CAD build for the part. Positions are in the model's coordinates, mm. Coordinates: 2 decimals unless noted, no trailing zeros. Order: outer loops, then holes, each group sorted by start corner. A loop starts at its lowest first (then second) coordinate and runs counter-clockwise, first axis right, second up. Notation, with made-up numbers: (57, -14.5) - (113, -14.5) arc R19 ccw to (113, 3.5) - close; hole circle Ø2 at (12.5, 63.5). An arc over 180 degrees is marked (long way). Use one line per item in the form item = value.
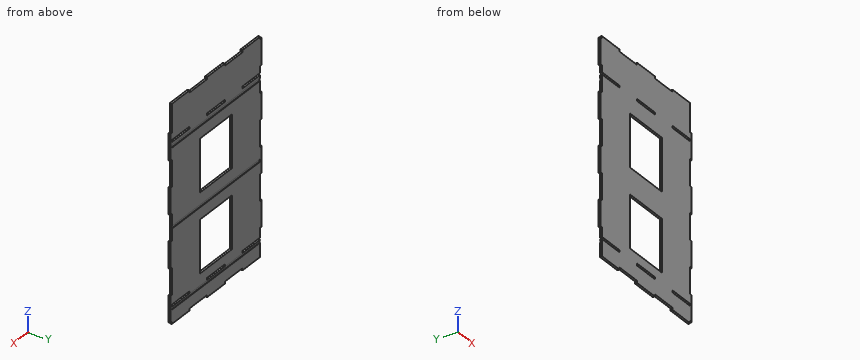
Autodesk Inventor part; units mm, degrees
ref_plane "YZ Plane" through (0, 0, 0) normal (1, 0, 0) x (0, 1, 0)
ref_plane "XZ Plane" through (0, 0, 0) normal (0, 1, 0) x (-1, 0, 0)
ref_plane "XY Plane" through (0, 0, 0) normal (0, 0, 1) x (1, 0, 0)
sketch "Sketch1" plane through (0, 0, 0) normal (0, 1, 0) x (-1, 0, 0)
  line L0 (-125, 200) -> (125, 200) construction
  line L1 (125, 200) -> (125, -200) construction
  line L2 (125, -200) -> (-125, -200) construction
  line L3 (-125, -200) -> (-125, 200) construction
  line L4 (-125, 200) -> (125, -200) construction
  line L5 (125, 200) -> (-125, -200) construction
  line L6 (125, 200) -> (75, 200) construction
  line L7 (75, 200) -> (75, 204)
  line L8 (75, 204) -> (125, 204)
  line L9 (125, 204) -> (125, 200)
  line L10 (125, 200) -> (129, 200)
  line L11 (129, 200) -> (129, 150)
  line L12 (129, 150) -> (125, 150)
  line L13 (125, 150) -> (125, 200) construction
  line L14 (-125, 200) -> (-129, 200) construction
  line L15 (-129, 200) -> (-129, 150) construction
  line L16 (-129, 150) -> (-125, 150)
  line L17 (-125, 150) -> (-125, 200)
  line L18 (125, -200) -> (75, -200) construction
  line L19 (75, -200) -> (75, -204)
  line L20 (75, -204) -> (125, -204)
  line L21 (125, -204) -> (125, -200)
  line L22 (125, 100) -> (125, 150)
  line L23 (125, 150) -> (129, 150)
  line L24 (129, 100) -> (125, 100)
  line L25 (129, 150) -> (129, 100) construction
  line L26 (-125, 100) -> (-125, 150) construction
  line L27 (-125, 150) -> (-129, 150)
  line L28 (-129, 150) -> (-129, 100)
  line L29 (-129, 100) -> (-125, 100)
  line L30 (125, 50) -> (125, 100) construction
  line L31 (125, 100) -> (129, 100)
  line L32 (129, 50) -> (125, 50)
  line L33 (129, 100) -> (129, 50)
  line L34 (-125, 50) -> (-125, 100)
  line L35 (-125, 100) -> (-129, 100)
  line L36 (-129, 100) -> (-129, 50) construction
  line L37 (-129, 50) -> (-125, 50)
  line L38 (125, 0) -> (125, 50)
  line L39 (125, 50) -> (129, 50)
  line L40 (129, 0) -> (125, 0)
  line L41 (129, 50) -> (129, 0) construction
  line L42 (-125, 0) -> (-125, 50) construction
  line L43 (-125, 50) -> (-129, 50)
  line L44 (-129, 50) -> (-129, 0)
  line L45 (-129, 0) -> (-125, 0)
  line L46 (125, -50) -> (125, 0) construction
  line L47 (125, 0) -> (129, 0)
  line L48 (129, -50) -> (125, -50)
  line L49 (129, 0) -> (129, -50)
  line L50 (-125, -50) -> (-125, 0)
  line L51 (-125, 0) -> (-129, 0)
  line L52 (-129, 0) -> (-129, -50) construction
  line L53 (-129, -50) -> (-125, -50)
  line L54 (125, -100) -> (125, -50)
  line L55 (125, -50) -> (129, -50)
  line L56 (129, -100) -> (125, -100)
  line L57 (129, -50) -> (129, -100) construction
  line L58 (-125, -100) -> (-125, -50) construction
  line L59 (-125, -50) -> (-129, -50)
  line L60 (-129, -50) -> (-129, -100)
  line L61 (-129, -100) -> (-125, -100)
  line L62 (125, -150) -> (125, -100) construction
  line L63 (125, -100) -> (129, -100)
  line L64 (129, -150) -> (125, -150)
  line L65 (129, -100) -> (129, -150)
  line L66 (-125, -150) -> (-125, -100)
  line L67 (-125, -100) -> (-129, -100)
  line L68 (-129, -100) -> (-129, -150) construction
  line L69 (-129, -150) -> (-125, -150)
  line L70 (125, -200) -> (125, -150)
  line L71 (125, -150) -> (129, -150)
  line L72 (129, -200) -> (125, -200) construction
  line L73 (129, -150) -> (129, -200) construction
  line L74 (-125, -200) -> (-125, -150) construction
  line L75 (-125, -150) -> (-129, -150)
  line L76 (-129, -150) -> (-129, -200)
  line L77 (-129, -200) -> (-125, -200)
  line L78 (75, 204) -> (75, 200)
  line L79 (25, 200) -> (25, 204)
  line L80 (25, 204) -> (75, 204) construction
  line L81 (75, 200) -> (25, 200)
  line L82 (75, -200) -> (25, -200)
  line L83 (25, -200) -> (25, -204)
  line L84 (25, -204) -> (75, -204) construction
  line L85 (75, -204) -> (75, -200)
  line L86 (25, 204) -> (25, 200)
  line L87 (-25, 200) -> (-25, 204)
  line L88 (-25, 204) -> (25, 204)
  line L89 (25, 200) -> (-25, 200) construction
  line L90 (25, -200) -> (-25, -200) construction
  line L91 (-25, -200) -> (-25, -204)
  line L92 (-25, -204) -> (25, -204)
  line L93 (25, -204) -> (25, -200)
  line L94 (-25, 204) -> (-25, 200)
  line L95 (-75, 200) -> (-75, 204)
  line L96 (-75, 204) -> (-25, 204) construction
  line L97 (-25, 200) -> (-75, 200)
  line L98 (-25, -200) -> (-75, -200)
  line L99 (-75, -200) -> (-75, -204)
  line L100 (-75, -204) -> (-25, -204) construction
  line L101 (-25, -204) -> (-25, -200)
  line L102 (-75, 204) -> (-75, 200)
  line L103 (-125, 200) -> (-125, 204)
  line L104 (-125, 204) -> (-75, 204)
  line L105 (-75, 200) -> (-125, 200) construction
  line L106 (-75, -200) -> (-125, -200) construction
  line L107 (-125, -200) -> (-125, -204)
  line L108 (-125, -204) -> (-75, -204)
  line L109 (-75, -204) -> (-75, -200)
  point P0 (0, 0)
  dimension "d0" = 250
  dimension "d1" = 400
  dimension "d2" = 50
  dimension "d3" = 4
  dimension "d4" = 4
  dimension "d5" = 50
  dimension "d6" = 4
  dimension "d7" = 50
  dimension "d8" = 50
  dimension "d9" = 4
  dimension "d12" = 50
  dimension "d19" = 50
extrude "Extrusion1" add sketch "Sketch1" along normal blind 4
sketch "Sketch2" plane through (0, 4, 0) normal (0, 1, 0) x (1, 0, 0)
  line L0 (-125, 100) -> (-125, 50)
  line L1 (129, 100) -> (125, 100)
  line L2 (-125, 100) -> (125, 100) construction
  line L3 (125, -100) -> (125, -50)
  line L4 (125, -50) -> (-125, -50) construction
  line L5 (-45, 150) -> (45, 150)
  line L6 (45, 150) -> (45, 50)
  line L7 (45, 50) -> (-45, 50)
  line L8 (-45, 50) -> (-45, 150)
  line L9 (-45, 150) -> (45, 50) construction
  line L10 (45, 150) -> (-45, 50) construction
  line L11 (45, -100) -> (-45, -100)
  line L12 (-45, -100) -> (-45, 0)
  line L13 (-45, 0) -> (45, 0)
  line L14 (45, 0) -> (45, -100)
  line L15 (45, -100) -> (-45, 0) construction
  line L16 (-45, -100) -> (45, 0) construction
  point P0 (0, 0)
  point P1 (0, 100)
  point P2 (0, -50)
  point P3 (0, -50)
  dimension "d26" = 90
  dimension "d27" = 100
  dimension "d28" = 90
  dimension "d29" = 100
extrude "Extrusion2" cut sketch "Sketch2" against normal up to next
sketch "Sketch3" plane through (0, 4, 0) normal (0, 1, 0) x (1, 0, 0)
  line L0 (-129, 50) -> (-129, 0)
  line L1 (125, 0) -> (125, 50)
  line L2 (-129, 27.5) -> (125, 27.5)
  line L3 (125, 27.5) -> (125, 22.5)
  line L4 (125, 22.5) -> (-129, 22.5)
  line L5 (-129, 22.5) -> (-129, 27.5)
  line L6 (-129, 25) -> (125, 25) construction
  line L7 (-129, 27.5) -> (-125, 27.5)
  line L8 (-125, 27.5) -> (-125, 22.5)
  line L9 (-125, 22.5) -> (-129, 22.5)
  line L10 (-129, 22.5) -> (-129, 27.5)
  line L11 (-125, 0) -> (-125, -50)
  point P0 (0, 0)
  point P1 (-125, 27.5)
  point P2 (-125, 22.5)
  dimension "d32" = 5
extrude "Extrusion3" cut sketch "Sketch3" against normal blind 1 contours L2 L1 L4 L8
sketch "Sketch4" plane through (0, 4, 0) normal (0, 1, 0) x (1, 0, 0)
  line L0 (-125, -127.5) -> (125, -127.5)
  line L1 (125, -127.5) -> (125, -122.5)
  line L2 (125, -122.5) -> (-125, -122.5)
  line L3 (-125, -122.5) -> (-125, -127.5)
  line L4 (-125, -127.5) -> (125, -122.5) construction
  line L5 (125, -127.5) -> (-125, -122.5) construction
  line L6 (-125, -100) -> (-125, -150)
  line L7 (-125, -125) -> (129, -125) construction
  line L8 (129, -150) -> (129, -100)
  line L9 (129, 150) -> (129, 200)
  line L10 (129, 175) -> (-125, 175) construction
  line L11 (-125, 204) -> (-125, 150)
  line L12 (-125, 172.5) -> (125, 172.5)
  line L13 (125, 172.5) -> (125, 177.5)
  line L14 (125, 177.5) -> (-125, 177.5)
  line L15 (-125, 177.5) -> (-125, 172.5)
  line L16 (-125, 172.5) -> (125, 177.5) construction
  line L17 (125, 172.5) -> (-125, 177.5) construction
  line L18 (125, 100) -> (125, 150)
  line L19 (-125, 204) -> (-125, 150)
  point P0 (0, 0)
  point P1 (0, -125)
  point P2 (125, -125)
  point P3 (125, -100)
  point P4 (-125, -125)
  point P5 (-125, 22.5)
  point P6 (0, 175)
  dimension "d36" = 5
  dimension "d39" = 5
extrude "Extrusion4" cut sketch "Sketch4" against normal blind 1
sketch "Sketch5" plane through (0, 4, 0) normal (0, 1, 0) x (1, 0, 0)
  line L0 (-125, -133) -> (-75, -133)
  line L1 (-75, -133) -> (-75, -137)
  line L2 (-75, -137) -> (-125, -137)
  line L3 (-125, -137) -> (-125, -133)
  line L4 (-75, -200) -> (-25, -200)
  line L5 (-125, -100) -> (-125, -122.5)
  line L6 (125, -127.5) -> (-125, -127.5)
  line L7 (-75, -133) -> (-25, -133)
  line L8 (-25, -133) -> (-25, -137)
  line L9 (-25, -137) -> (-75, -137)
  line L10 (-75, -137) -> (-75, -133)
  line L11 (-25, -133) -> (25, -133)
  line L12 (25, -133) -> (25, -137)
  line L13 (25, -137) -> (-25, -137)
  line L14 (-25, -137) -> (-25, -133)
  line L15 (25, -133) -> (75, -133)
  line L16 (75, -133) -> (75, -137)
  line L17 (75, -137) -> (25, -137)
  line L18 (25, -137) -> (25, -133)
  line L19 (75, -133) -> (125, -133)
  line L20 (125, -133) -> (125, -137)
  line L21 (125, -137) -> (75, -137)
  line L22 (75, -137) -> (75, -133)
  line L23 (-25, 168) -> (-75, 168)
  line L24 (-75, 172) -> (-25, 172)
  line L25 (-25, 172) -> (-25, 168)
  line L26 (-25, 168) -> (-25, 172)
  line L27 (25, 168) -> (-25, 168)
  line L28 (-25, 172) -> (25, 172)
  line L29 (25, 172) -> (25, 168)
  line L30 (25, 168) -> (25, 172)
  line L31 (25, 172) -> (75, 172)
  line L32 (75, 168) -> (25, 168)
  line L33 (-75, 172) -> (-75, 168)
  line L34 (-75, 168) -> (-75, 172)
  line L35 (-125, 172) -> (-75, 172)
  line L36 (-125, 168) -> (-125, 172)
  line L37 (-75, 168) -> (-125, 168)
  line L38 (75, 172) -> (75, 168)
  line L39 (75, 168) -> (75, 172)
  line L40 (75, 172) -> (125, 172)
  line L41 (125, 172) -> (125, 168)
  line L42 (125, 168) -> (75, 168)
  point P0 (0, 0)
  dimension "d40" = 50
  dimension "d41" = 4
  dimension "d42" = 63
  dimension "d45" = 50
  dimension "d54" = 305
extrude "Extrusion5" cut sketch "Sketch5" against normal up to next contours L0 L1 L2 L3 | L11 L12 L13 L8 | L19 L20 L21 L16 | L25 L28 L29 L27 | L37 L36 L35 L33 | L38 L40 L41 L42
properties part number "DoorFront_V1"
Item 1: Cut at B-B, the plane z = 63. Write the cut outline in (x, y), plus the area to 3 significant figures.
Derived:
outline = (-129, 0) - (-45, 0) - (-45, 4) - (-129, 4) - close; (45, 0) - (125, 0) - (125, 4) - (45, 4) - close
area = 656 mm²
Item 2: Drill centre lines: line 1 (Z direction, x = -76.5, y = 2.9); line 2 (Z direction, x = -110, y = 3.65); line 3 (X direction, y = 2.05, z = 135.5). Where is each one in solid material? Low to high. Write a range as [from, to].
Derived:
line_1 = [-204, -172], [-168, 133], [137, 204]
line_2 = [-204, -177.5], [-172.5, -172], [-168, -27.5], [-22.5, 122.5], [127.5, 133], [137, 204]
line_3 = [-75, -25], [25, 75], [125, 129]
Item 3: Cut at A-A, the plane x = -0.5. State how many separate pieces and enclosed holes the cut face has, plus the area to 3 significant figures.
Derived:
separate_pieces = 5
enclosed_holes = 0
area = 785 mm²
Item 4: Cut at C-C, the plane x = -63.5. Write the cut outline in (y, z).
Derived:
outline = (0, -200) - (4, -200) - (4, -177.5) - (3, -177.5) - (3, -172.5) - (4, -172.5) - (4, -27.5) - (3, -27.5) - (3, -22.5) - (4, -22.5) - (4, 122.5) - (3, 122.5) - (3, 127.5) - (4, 127.5) - (4, 200) - (0, 200) - close
Item 5: Drop flat-ended pins along their axis: pin 1 (1 mm diameter, centred on x = -71, y = 1.5, fed in from -Z); pin 2 (0.5 mm diameter, centred on x = 58.5, y = 3.5, fed in from +Z); pin 3 (10 mm diameter, centred on x = -25, z = 114.5, fed in from -Y); pin 4 (2 mm diameter, centred on y = 1.5, z = -27.5, fed in from +X). Give the stop position or say it passes through.
Derived:
pin_1 = -200
pin_2 = 200
pin_3 = 0
pin_4 = 125
